```python
from build123d import *

# Parameters (mm, degrees)
SKETCH1_R           = 1.7859375
BOSS_EXTRUDE1_DEPTH = 0.8128


with BuildPart() as part:
    # Sketch1 → Boss-Extrude1 (new body)
    with BuildSketch(Plane.XY):
        with BuildLine():
            ThreePointArc((5.113201945, -2.174184888), (6.429738065, -0.592725341), (8.400260413, 0))
            Line((8.400260413, 0), (32.874739587, 0))
            ThreePointArc((32.874739587, 0), (34.845261898, -0.592725316), (36.161798019, -2.174184805))
            ThreePointArc((36.161798019, -2.174184805), (39.929142732, -5.390786796), (44.766280182, -4.322369345))
            ThreePointArc((44.766280182, -4.322369345), (46.671647173, -3.545286328), (48.689532151, -3.948301971))
            ThreePointArc((48.689532151, -3.948301971), (52.071763604, -3.935123969), (53.926672666, -1.106877933))
            ThreePointArc((53.926672666, -1.106877933), (50.638422177, 8.579995637), (41.275, 12.7))
            Line((41.275, 12.7), (34.13125, 12.7))
            ThreePointArc((34.13125, 12.7), (31.605552966, 11.653822034), (30.559375, 9.128125))
            ThreePointArc((30.559375, 9.128125), (29.513197034, 6.602427966), (26.9875, 5.55625))
            Line((26.9875, 5.55625), (14.2875, 5.55625))
            ThreePointArc((14.2875, 5.55625), (11.761802966, 6.602427966), (10.715625, 9.128125))
            ThreePointArc((10.715625, 9.128125), (9.669447034, 11.653822034), (7.14375, 12.7))
            Line((7.14375, 12.7), (0, 12.7))
            ThreePointArc((0, 12.7), (-9.363422177, 8.579995637), (-12.651672666, -1.106877933))
            ThreePointArc((-12.651672666, -1.106877933), (-10.796763578, -3.935123983), (-7.414532098, -3.948301943))
            ThreePointArc((-7.414532098, -3.948301943), (-5.396647132, -3.545286332), (-3.491280162, -4.322369361))
            ThreePointArc((-3.491280162, -4.322369361), (1.345857236, -5.390786804), (5.113201945, -2.174184888))
        make_face()
        with BuildLine():
            ThreePointArc((52.147531197, -0.951223224), (50.212735019, -2.574709983), (48.58924826, -0.639913805))
            ThreePointArc((48.58924826, -0.639913805), (46.688228446, 4.960309977), (41.275, 7.3421875))
            ThreePointArc((41.275, 7.3421875), (39.4890625, 9.128125), (41.275, 10.9140625))
            ThreePointArc((41.275, 10.9140625), (49.321690934, 7.37343375), (52.147531197, -0.951223224))
        make_face(mode=Mode.SUBTRACT)
        with BuildLine():
            ThreePointArc((0, 10.9140625), (1.7859375, 9.128125), (0, 7.3421875))
            ThreePointArc((0, 7.3421875), (-5.413228446, 4.960309977), (-7.31424826, -0.639913805))
            ThreePointArc((-7.31424826, -0.639913805), (-8.937735019, -2.574709983), (-10.872531197, -0.951223224))
            ThreePointArc((-10.872531197, -0.951223224), (-8.046690934, 7.37343375), (0, 10.9140625))
        make_face(mode=Mode.SUBTRACT)
        Circle(SKETCH1_R, mode=Mode.SUBTRACT)
        with Locations((41.275, 0)):
            Circle(SKETCH1_R, mode=Mode.SUBTRACT)
        with Locations((7.14375, 9.128125)):
            Circle(SKETCH1_R, mode=Mode.SUBTRACT)
        with Locations((34.13125, 9.128125)):
            Circle(SKETCH1_R, mode=Mode.SUBTRACT)
    extrude(amount=BOSS_EXTRUDE1_DEPTH)


solid = part.part
```
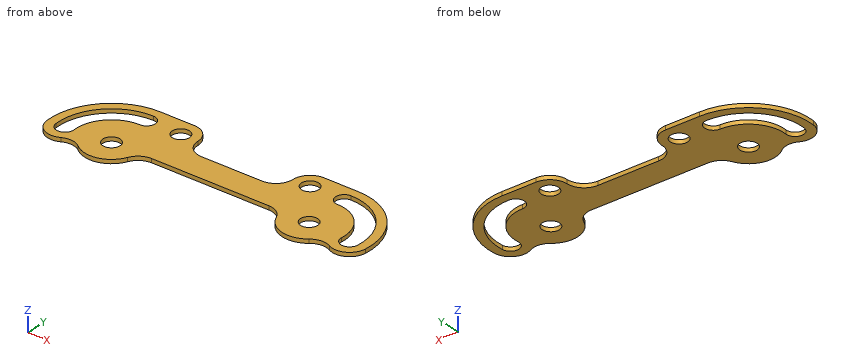
For this review, take the finished solid that the model builds, in its own axes (mm). Coordinates: 2 decimals unless noted, no trailing zeros. Loops run counter-clockwise (first coordinate to the right, second up) from the corner with the lowest first, then second, coordinate; pieces in that order, holes last. Notation, with made-up numbers: (80, -37) - (137, -37) arc R30 ccw to (137, -11) - close; hole circle Ø7 at (23, 2). An arc over 180 degrees is marked (long way). Use one line per item in the form item = value. Start each with the question number.
1) To check wall thickness, follow probe 1 along X at (y, z) = (0.75, 0.7); probe 2 along X at (y, z) = (5, 0.75); probe 3 along X at (y, z) = (2.25, 0.5). State the ranges of each line that lie inside material, in increasing order. Write a range as from..to.
2) Take a section at D-D (x = 20). State the section outline as (y, z) points, plus the area to 3 significant figures.
3) Take a section at A-A (x = 35). State the section outline as (y, z) points, plus the area to 3 significant figures.
4) Take a section at B-B (z = 0.25). State how many separate pieces and enclosed holes the cut face has, plus the area to 3 significant figures.
5) Take a section at C-C (y = 3.75). State the section outline as (x, z) points, plus the area to 3 significant figures.
6) For pin 1 (2 mm diameter, centred on x = 41.275, y = 0, fed in from +Z), flat-tipped, find the tip position at first contact; note if it passes through.
From the geometry:
q1.probe_1 = -12.68..-10.89, -7.3..-1.62, 1.62..39.65, 42.9..48.58, 52.16..53.95
q1.probe_2 = -11.67..-9.7, -5.38..46.65, 50.98..52.95
q1.probe_3 = -12.5..-10.68, -6.99..48.26, 51.95..53.77
q2.outline = (0, 0) - (5.56, 0) - (5.56, 0.81) - (0, 0.81) - close
q2.area = 4.52 mm2
q3.outline = (-0.7, 0) - (7.57, 0) - (7.57, 0.81) - (-0.7, 0.81) - close; (10.69, 0) - (12.7, 0) - (12.7, 0.81) - (10.69, 0.81) - close
q3.area = 8.36 mm2
q4.separate_pieces = 1
q4.enclosed_holes = 6
q4.area = 624 mm2
q5.outline = (-12.13, 0) - (-10.25, 0) - (-10.25, 0.81) - (-12.13, 0.81) - close; (-6.31, 0) - (47.59, 0) - (47.59, 0.81) - (-6.31, 0.81) - close; (51.52, 0) - (53.41, 0) - (53.41, 0.81) - (51.52, 0.81) - close
q5.area = 46.9 mm2
q6.pin_1 = through
